Check sheet for the modelled part. Datum: model origin and axes. Units: mm. A direction names the side the tool comes from. Coordinates: 2 decimals unless noted, no trailing zeros. Loops run counter-clockwise (first coordinate to the right, second up) from the corner with the lowest first, then second, coordinate; pieces in that order, holes last. Notation, with made-up numbers: (72.5, 45) -> (127.5, 45) arc R25 ccw to (127.5, 72) -> close; hole circle Ø8 at (8, 74). An arc over 180 degrees is marked (long way). Use one line per item in the form item = value.
from build123d import *

# Parameters (mm, degrees)
SKETCH_1_W           = 78.5
SKETCH_1_H           = 52
EXTRUDE_1_DEPTH      = 150
SKETCH_2_W           = 42
SKETCH_2_H           = 42
CUT_EXTRUDE_1_DEPTH  = 38
SKETCH_3_R           = 18
CUT_EXTRUDE_2_DEPTH  = 38.5
CUT_EXTRUDE_3_REACH  = 172.377
SKETCH_4_R           = 11
CUT_EXTRUDE_4_REACH  = 173.284
SKETCH_5_R           = 1.5
CUT_EXTRUDE_5_REACH  = 173.284
SKETCH_8_R           = 1.5
SKETCH_15_W          = 42
SKETCH_15_H          = 88
CUT_EXTRUDE_13_DEPTH = 20
SKETCH_16_R          = 11
CUT_EXTRUDE_14_DEPTH = 2
SKETCH_17_R          = 18
CUT_EXTRUDE_15_DEPTH = 27.5
SKETCH_18_W          = 42
SKETCH_18_H          = 42
SKETCH_18_R          = 18
SKETCH_18_R_2        = 11
CUT_EXTRUDE_16_DEPTH = 29
CUT_EXTRUDE_17_REACH = 165.09
SKETCH_19_R          = 1.5


with BuildPart() as part:
    # 草图1 → 凸台-拉伸1 (new body)
    with BuildSketch(Plane(origin=(0, 0, 0), x_dir=(1, 0, 0), z_dir=(0, 1, 0))):
        Rectangle(SKETCH_1_W, SKETCH_1_H)
    extrude(amount=EXTRUDE_1_DEPTH)

    # 草图2 → 切除-拉伸1 (cut)
    with BuildSketch(Plane.ZY.offset(39.25)):
        with Locations((0, 26)):
            Rectangle(SKETCH_2_W, SKETCH_2_H)
    extrude(amount=-CUT_EXTRUDE_1_DEPTH, mode=Mode.SUBTRACT)

    # 草图3 → 切除-拉伸2 (cut)
    with BuildSketch(Plane.ZY.offset(1.25)):
        with Locations((0, 26)):
            Circle(SKETCH_3_R)
    extrude(amount=-CUT_EXTRUDE_2_DEPTH, mode=Mode.SUBTRACT)

    # 草图4 → 切除-拉伸3 (cut, up to next)
    with BuildSketch(Plane.ZY.offset(-37.25), mode=Mode.PRIVATE) as cut_extrude_3_sk1:
        with Locations((0, 26)):
            Circle(SKETCH_4_R)
    cut_extrude_3_tool1 = extrude(cut_extrude_3_sk1.sketch, amount=-CUT_EXTRUDE_3_REACH, mode=Mode.PRIVATE) & part.part
    add(cut_extrude_3_tool1.solids().sort_by_distance((37.25, 26, 0))[0], mode=Mode.SUBTRACT)

    # 草图5 → 切除-拉伸4 (cut, up to next)
    with BuildSketch(Plane(origin=(39.25, 0, 0), x_dir=(0, 0, -1), z_dir=(1, 0, 0)), mode=Mode.PRIVATE) as cut_extrude_4_sk1:
        with Locations((-9.899494937, 35.899494937)):
            Circle(SKETCH_5_R)
    cut_extrude_4_tool1 = extrude(cut_extrude_4_sk1.sketch, amount=-CUT_EXTRUDE_4_REACH, mode=Mode.PRIVATE) & part.part
    # 草图5 → 切除-拉伸4 (cut, up to next)
    with BuildSketch(Plane(origin=(39.25, 0, 0), x_dir=(0, 0, -1), z_dir=(1, 0, 0)), mode=Mode.PRIVATE) as cut_extrude_4_sk2:
        with Locations((9.899494937, 35.899494937)):
            Circle(SKETCH_5_R)
    cut_extrude_4_tool2 = extrude(cut_extrude_4_sk2.sketch, amount=-CUT_EXTRUDE_4_REACH, mode=Mode.PRIVATE) & part.part
    # 草图5 → 切除-拉伸4 (cut, up to next)
    with BuildSketch(Plane(origin=(39.25, 0, 0), x_dir=(0, 0, -1), z_dir=(1, 0, 0)), mode=Mode.PRIVATE) as cut_extrude_4_sk3:
        with Locations((9.899494937, 16.100505063)):
            Circle(SKETCH_5_R)
    cut_extrude_4_tool3 = extrude(cut_extrude_4_sk3.sketch, amount=-CUT_EXTRUDE_4_REACH, mode=Mode.PRIVATE) & part.part
    # 草图5 → 切除-拉伸4 (cut, up to next)
    with BuildSketch(Plane(origin=(39.25, 0, 0), x_dir=(0, 0, -1), z_dir=(1, 0, 0)), mode=Mode.PRIVATE) as cut_extrude_4_sk4:
        with Locations((-9.899494937, 16.100505063)):
            Circle(SKETCH_5_R)
    cut_extrude_4_tool4 = extrude(cut_extrude_4_sk4.sketch, amount=-CUT_EXTRUDE_4_REACH, mode=Mode.PRIVATE) & part.part
    add(cut_extrude_4_tool1.solids().sort_by_distance((39.25, 35.899495, 9.899495))[0], mode=Mode.SUBTRACT)
    add(cut_extrude_4_tool2.solids().sort_by_distance((39.25, 35.899495, -9.899495))[0], mode=Mode.SUBTRACT)
    add(cut_extrude_4_tool3.solids().sort_by_distance((39.25, 16.100505, -9.899495))[0], mode=Mode.SUBTRACT)
    add(cut_extrude_4_tool4.solids().sort_by_distance((39.25, 16.100505, 9.899495))[0], mode=Mode.SUBTRACT)

    # 草图8 → 切除-拉伸5 (cut, up to next)
    with BuildSketch(Plane(origin=(39.25, 0, 0), x_dir=(0, 0, -1), z_dir=(1, 0, 0)), mode=Mode.PRIVATE) as cut_extrude_5_sk1:
        with Locations((-15.5, 41.5)):
            Circle(SKETCH_8_R)
    cut_extrude_5_tool1 = extrude(cut_extrude_5_sk1.sketch, amount=-CUT_EXTRUDE_5_REACH, mode=Mode.PRIVATE) & part.part
    # 草图8 → 切除-拉伸5 (cut, up to next)
    with BuildSketch(Plane(origin=(39.25, 0, 0), x_dir=(0, 0, -1), z_dir=(1, 0, 0)), mode=Mode.PRIVATE) as cut_extrude_5_sk2:
        with Locations((15.5, 41.5)):
            Circle(SKETCH_8_R)
    cut_extrude_5_tool2 = extrude(cut_extrude_5_sk2.sketch, amount=-CUT_EXTRUDE_5_REACH, mode=Mode.PRIVATE) & part.part
    # 草图8 → 切除-拉伸5 (cut, up to next)
    with BuildSketch(Plane(origin=(39.25, 0, 0), x_dir=(0, 0, -1), z_dir=(1, 0, 0)), mode=Mode.PRIVATE) as cut_extrude_5_sk3:
        with Locations((-15.5, 10.5)):
            Circle(SKETCH_8_R)
    cut_extrude_5_tool3 = extrude(cut_extrude_5_sk3.sketch, amount=-CUT_EXTRUDE_5_REACH, mode=Mode.PRIVATE) & part.part
    # 草图8 → 切除-拉伸5 (cut, up to next)
    with BuildSketch(Plane(origin=(39.25, 0, 0), x_dir=(0, 0, -1), z_dir=(1, 0, 0)), mode=Mode.PRIVATE) as cut_extrude_5_sk4:
        with Locations((15.5, 10.5)):
            Circle(SKETCH_8_R)
    cut_extrude_5_tool4 = extrude(cut_extrude_5_sk4.sketch, amount=-CUT_EXTRUDE_5_REACH, mode=Mode.PRIVATE) & part.part
    add(cut_extrude_5_tool1.solids().sort_by_distance((39.25, 41.5, 15.5))[0], mode=Mode.SUBTRACT)
    add(cut_extrude_5_tool2.solids().sort_by_distance((39.25, 41.5, -15.5))[0], mode=Mode.SUBTRACT)
    add(cut_extrude_5_tool3.solids().sort_by_distance((39.25, 10.5, 15.5))[0], mode=Mode.SUBTRACT)
    add(cut_extrude_5_tool4.solids().sort_by_distance((39.25, 10.5, -15.5))[0], mode=Mode.SUBTRACT)

    # 草图15 → 切除-拉伸13 (cut)
    with BuildSketch(Plane.ZY.offset(39.25)):
        with Locations((0, 101)):
            Rectangle(SKETCH_15_W, SKETCH_15_H)
    extrude(amount=-CUT_EXTRUDE_13_DEPTH, mode=Mode.SUBTRACT)

    # 草图16 → 切除-拉伸14 (cut)
    with BuildSketch(Plane.ZY.offset(19.25)):
        with Locations((0, 78)):
            Circle(SKETCH_16_R)
    extrude(amount=-CUT_EXTRUDE_14_DEPTH, mode=Mode.SUBTRACT)

    # 草图17 → 切除-拉伸15 (cut)
    with BuildSketch(Plane.ZY.offset(17.25)):
        with Locations((0, 78)):
            Circle(SKETCH_17_R)
    extrude(amount=-CUT_EXTRUDE_15_DEPTH, mode=Mode.SUBTRACT)

    # 草图18 → 切除-拉伸16 (cut)
    # profile 1 of 3: a face of its own
    with BuildSketch(Plane.ZY.offset(-10.25)):
        with Locations((0, 78)):
            Rectangle(SKETCH_18_W, SKETCH_18_H)
        with Locations((0, 78)):
            Circle(SKETCH_18_R, mode=Mode.SUBTRACT)
    # profile 2 of 3: a face of its own
    with BuildSketch(Plane.ZY.offset(-10.25)):
        with Locations((0, 78)):
            Circle(SKETCH_18_R)
        with Locations((0, 78)):
            Circle(SKETCH_18_R_2, mode=Mode.SUBTRACT)
    # profile 3 of 3: a face of its own
    with BuildSketch(Plane.ZY.offset(-10.25)):
        with Locations((0, 78)):
            Circle(SKETCH_18_R_2)
    extrude(amount=-CUT_EXTRUDE_16_DEPTH, mode=Mode.SUBTRACT)

    # 草图19 → 切除-拉伸17 (cut, up to next)
    with BuildSketch(Plane.ZY.offset(19.25), mode=Mode.PRIVATE) as cut_extrude_17_sk1:
        with Locations((-9.899494937, 87.899494937)):
            Circle(SKETCH_19_R)
    cut_extrude_17_tool1 = extrude(cut_extrude_17_sk1.sketch, amount=-CUT_EXTRUDE_17_REACH, mode=Mode.PRIVATE) & part.part
    # 草图19 → 切除-拉伸17 (cut, up to next)
    with BuildSketch(Plane.ZY.offset(19.25), mode=Mode.PRIVATE) as cut_extrude_17_sk2:
        with Locations((9.899494937, 87.899494937)):
            Circle(SKETCH_19_R)
    cut_extrude_17_tool2 = extrude(cut_extrude_17_sk2.sketch, amount=-CUT_EXTRUDE_17_REACH, mode=Mode.PRIVATE) & part.part
    # 草图19 → 切除-拉伸17 (cut, up to next)
    with BuildSketch(Plane.ZY.offset(19.25), mode=Mode.PRIVATE) as cut_extrude_17_sk3:
        with Locations((9.899494937, 68.100505063)):
            Circle(SKETCH_19_R)
    cut_extrude_17_tool3 = extrude(cut_extrude_17_sk3.sketch, amount=-CUT_EXTRUDE_17_REACH, mode=Mode.PRIVATE) & part.part
    # 草图19 → 切除-拉伸17 (cut, up to next)
    with BuildSketch(Plane.ZY.offset(19.25), mode=Mode.PRIVATE) as cut_extrude_17_sk4:
        with Locations((-9.899494937, 68.100505063)):
            Circle(SKETCH_19_R)
    cut_extrude_17_tool4 = extrude(cut_extrude_17_sk4.sketch, amount=-CUT_EXTRUDE_17_REACH, mode=Mode.PRIVATE) & part.part
    add(cut_extrude_17_tool1.solids().sort_by_distance((-19.25, 87.899495, -9.899495))[0], mode=Mode.SUBTRACT)
    add(cut_extrude_17_tool2.solids().sort_by_distance((-19.25, 87.899495, 9.899495))[0], mode=Mode.SUBTRACT)
    add(cut_extrude_17_tool3.solids().sort_by_distance((-19.25, 68.100505, 9.899495))[0], mode=Mode.SUBTRACT)
    add(cut_extrude_17_tool4.solids().sort_by_distance((-19.25, 68.100505, -9.899495))[0], mode=Mode.SUBTRACT)


solid = part.part
(1) Mould release check, pull along Z, two halves, no side actions. Record for faces 1 (the cylindrical face through (38.24, 15.26, -2.38)), 2 (the flat face through (-1, 74, -26)), 3 (the flat face through (-1, 150, 0)): +Z half, -Z half, draft (parallel to the pull), parting line (faces both ways), or undercut.
Established:
face_1 = undercut
face_2 = -Z half
face_3 = draft
(2) Scan lines: line 1 along Y through (x, z) = (38.1, 0); line 2 along Y through (x, z) = (-28.5, -7.5); line 3 along Z through (x, y) = (-25.5, 25.5). Record each from-to range of solid material in increasing order.
Established:
line_1 = 0 to 15, 37 to 57, 99 to 150
line_2 = 0 to 5, 47 to 57, 145 to 150
line_3 = -26 to -21, 21 to 26
(3) Section check D-D, the plane y = 105. Record the boundary of the cut face in (x, z).
Established:
outline = (-39.25, -26) -> (39.25, -26) -> (39.25, 26) -> (-39.25, 26) -> (-39.25, 21) -> (-19.25, 21) -> (-19.25, -21) -> (-39.25, -21) -> close
(4) Section check A-A, the plane x = 33.5. Record the boundary of the cut face in (y, z), plus the area to 3 significant figures.
Established:
outline = (0, -26) -> (150, -26) -> (150, 26) -> (0, 26) -> close; hole circle Ø36 at (26, 0); hole circle Ø3 at (10.5, -15.5); hole circle Ø3 at (10.5, 15.5); hole circle Ø3 at (41.5, -15.5); hole circle Ø3 at (41.5, 15.5); hole (57, -21) -> (99, -21) -> (99, 21) -> (57, 21) -> close
area = 4,990 mm²
(5) Section check C-C, the plane z = 4.5. Give the number of separate pieces and of enclosed holes in the cut face, plus the area to 3 significant figures.
Established:
separate_pieces = 3
enclosed_holes = 0
area = 4,820 mm²
(6) Section check B-B, the plane y = 10.5. Record the boundary of the cut face in (x, z), plus the area to 3 significant figures.
Established:
outline = (-39.25, -26) -> (39.25, -26) -> (39.25, -17) -> (-1.25, -17) -> (-1.25, -21) -> (-39.25, -21) -> close; (-39.25, 21) -> (-1.25, 21) -> (-1.25, 17) -> (39.25, 17) -> (39.25, 26) -> (-39.25, 26) -> close; (-1.25, -14) -> (39.25, -14) -> (39.25, 14) -> (-1.25, 14) -> (-1.25, 9.15) -> (37.25, 9.15) -> (37.25, -9.15) -> (-1.25, -9.15) -> close
area = 1,540 mm²
(7) Go/stop test with a flat-tipped pin: P1, Ø5, axis at y = 68.1, z = -9.9, coming from the -X side. Record where the tip stops, or that it passes through.
Established:
P1 = -19.25
(8) Tool access check on faces 4 (the flat face through (-1, 0, 0)), 5 (the flat face through (-17.25, 70, -8)), 6 (the flat face through (-21, 5, 0)). Record the directions out of +Z, -Z, +X, -X, +Y, -Y that give a thin tool (end or side, any length) a straight path to the whole face; none if there is none.
Established:
face_4 = +Z, -Z, +X, -X, -Y
face_5 = +X
face_6 = -X
